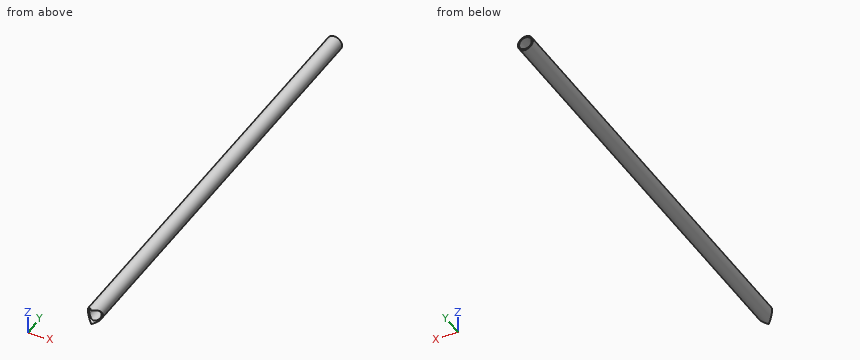
Solid Edge part; units mm, degrees
sketch "Sketch1" plane through (0, 0, 0) normal (0, 0, 1) x (1, 0, 0)
  line L0 (0, 0) -> (0, 736.96)
sketch "Sketch2" plane through (0, 0, 0) normal (0, -1, 0) x (1, 0, 0)
  circle A0 centre (0, 0) radius 12.5
sweep "SweptProtrusion_1" add profiles "Sketch2" path "Sketch1"
shell "Thinwall_1" thickness 2 removed faces 2 at (-8.0833, 0, 8.5833) at (-8.0833, 736.96, 8.5833)
sketch "Sketch3" plane through (0, 0, 0) normal (1, 0, 0) x (0, 1, 0)
  circle A0 centre (0, 0) radius 12.5
extrude "Cutout1" cut sketch "Sketch3" along normal through all and the other way through all
properties material "Stainless steel"
Design review of the part built by this model. Coordinates are the model's own, in mm. Give positions to 0.01 mm unless a question says otherwise; leave off trailing zeros. Write each loop counter-clockwise with the first axis right and the second up, starting at its lowest first coordinate (ties: lowest second). Pieces come first, ordered by that corner, then holes.
(1) Clearance check with flat-ended pins moving along their axes: pin 1 Ø8 at (y, z) = (578.5, -5.5) entering from +X; pin 2 Ø2 at (y, z) = (83, -9.5) entering from +X; pin 3 Ø1.5 at (y, z) = (242.5, 8) entering from +X. State where each tip first meets the part, or that it passes through.
Checked values:
pin 1: stops at x = 12.41
pin 2: stops at x = 9.17
pin 3: stops at x = 10.18
(2) Add section B-B (x = 5). Give the boundary of the cut face in (y, z).
Checked values:
outline: (5, -11.46) - (736.96, -11.46) - (736.96, -9.23) - (8.43, -9.23) arc R12.5 cw to start; (5, 11.46) arc R12.5 cw to (8.43, 9.23) - (736.96, 9.23) - (736.96, 11.46) - close
(3) Wall thickness on line 1 along Z through (x, y) = (0, 293); line 2 along Y through (x, z) = (-8.5, 6.75); line 3 along X through (y, z) = (396, -1.5): over which ranges is each line inside the solid? List them lowest first.
Checked values:
line 1: z = -12.5 to -10.5, 10.5 to 12.5
line 2: y = 10.52 to 736.96
line 3: x = -12.41 to -10.39, 10.39 to 12.41
(4) Add section A-A (z = 0). Give the boundary of the cut face in (x, y), and give its area (3 significant figures).
Checked values:
outline: (-12.5, 12.5) - (-10.5, 12.5) - (-10.5, 736.96) - (-12.5, 736.96) - close; (10.5, 12.5) - (12.5, 12.5) - (12.5, 736.96) - (10.5, 736.96) - close
area: 2,900 mm2
(5) Add section C-C (y = 68). Give the boundary of the cut face in (x, z).
Checked values:
outline: circle Ø25 at (0, 0); hole circle Ø21 at (0, 0)
